Geometry: final body of the model. Coordinates: model frame, mm. A direction names the side the tool comes from. Give positions to 0.01 mm unless a question says otherwise; leave off trailing zeros. Order: outer loops, then holes, each group sorted by start corner. A loop starts at its lowest first (then second) coordinate and runs counter-clockwise, first axis right, second up. Notation, with made-up numbers: M 10.25,27.5 L 38.25,27.5 A19 ccw 38.25,36.5 Z; hole C 88.5,-29.75 d11. An arc over 180 degrees is marked long. One line per item, written item: value. Start each with the question number.
```python
from build123d import *

# Parameters (mm, degrees)
SKETCH1_R                    = 6.349999995
SKETCH1_R_2                  = 2.75
SKETCH1_R_3                  = 2.999999999
SKETCH1_R_4                  = 20
BOSS_EXTRUDE1_DEPTH          = 4.7625
FILLET1_R                    = 5.08
M5_TAPPED_HOLE1_D            = 4.2
M5_TAPPED_HOLE1_DEPTH        = 14
M5_TAPPED_HOLE1_TIP          = 1.2618073
F_3_0_3_DIAMETER_HOLE1_D     = 3
F_3_0_3_DIAMETER_HOLE1_DEPTH = 25.4
F_3_0_3_DIAMETER_HOLE1_TIP   = 0.901290929


with BuildPart() as part:
    # Sketch1 → Boss-Extrude1 (new body)
    # profile 1 of 6: a face of its own
    with BuildSketch(Plane.XY):
        Polygon((0, 57.15), (0, 0), (-8.945, -2.86), (-8.945, -40), (8.575, -40), (48.575, -40), (57.15, 0), (57.15, 57.15), align=None)
        with Locations(Location((-0.185, -21.43, 0), (0, 0, 180))):
            Circle(SKETCH1_R, mode=Mode.SUBTRACT)
        with Locations((4.953, 4.989071325)):
            Circle(SKETCH1_R_2, mode=Mode.SUBTRACT)
        with Locations(Location((28.575, -31.5, 0), (0, 0, 180))):
            Circle(SKETCH1_R_3, mode=Mode.SUBTRACT)
        with Locations(Location((28.575, -11.5, 0), (0, 0, 180))):
            Circle(SKETCH1_R_3, mode=Mode.SUBTRACT)
        with Locations((52.197, 4.989071325)):
            Circle(SKETCH1_R_2, mode=Mode.SUBTRACT)
        with Locations((4.953, 52.233071325)):
            Circle(SKETCH1_R_2, mode=Mode.SUBTRACT)
        with Locations(Location((28.575, 28.575, 0), (0, 0, 180))):
            Circle(SKETCH1_R_4, mode=Mode.SUBTRACT)
        with Locations((52.197, 52.197)):
            Circle(SKETCH1_R_2, mode=Mode.SUBTRACT)
    # profile 2 of 6: a face of its own
    with BuildSketch(Plane.XY):
        Polygon((0, 57.15), (0, 0), (-8.945, -2.86), (-8.945, -40), (8.575, -40), (48.575, -40), (57.15, 0), (57.15, 57.15), align=None)
        with Locations(Location((-0.185, -21.43, 0), (0, 0, 180))):
            Circle(SKETCH1_R, mode=Mode.SUBTRACT)
        with Locations((4.953, 4.989071325)):
            Circle(SKETCH1_R_2, mode=Mode.SUBTRACT)
        with Locations(Location((28.575, -31.5, 0), (0, 0, 180))):
            Circle(SKETCH1_R_3, mode=Mode.SUBTRACT)
        with Locations(Location((28.575, -11.5, 0), (0, 0, 180))):
            Circle(SKETCH1_R_3, mode=Mode.SUBTRACT)
        with Locations((52.197, 4.989071325)):
            Circle(SKETCH1_R_2, mode=Mode.SUBTRACT)
        with Locations((4.953, 52.233071325)):
            Circle(SKETCH1_R_2, mode=Mode.SUBTRACT)
        with Locations(Location((28.575, 28.575, 0), (0, 0, 180))):
            Circle(SKETCH1_R_4, mode=Mode.SUBTRACT)
        with Locations((52.197, 52.197)):
            Circle(SKETCH1_R_2, mode=Mode.SUBTRACT)
    # profile 3 of 6: a face of its own
    with BuildSketch(Plane.XY):
        with Locations((4.953, 52.233071325)):
            Circle(SKETCH1_R_2)
    # profile 4 of 6: a face of its own
    with BuildSketch(Plane.XY):
        with Locations((52.197, 52.197)):
            Circle(SKETCH1_R_2)
    # profile 5 of 6: a face of its own
    with BuildSketch(Plane.XY):
        with Locations((4.953, 4.989071325)):
            Circle(SKETCH1_R_2)
    # profile 6 of 6: a face of its own
    with BuildSketch(Plane.XY):
        with Locations((52.197, 4.989071325)):
            Circle(SKETCH1_R_2)
    extrude(amount=BOSS_EXTRUDE1_DEPTH)

    # Fillet1
    fillet1_edges = [part.edges().sort_by_distance(p)[0] for p in [
        (-8.945, -40, 2.38125),
        (-8.945, -2.86, 2.38125),
        (0, 0, 2.38125),
        (0, 57.15, 2.38125),
        (57.15, 57.15, 2.38125),
        (57.15, 0, 2.38125),
        (48.575, -40, 2.38125),
    ]]
    fillet(fillet1_edges, radius=FILLET1_R)

    # M5 Tapped Hole1
    with Locations(Plane.XY.offset(4.7625)):
        with Locations((4.953, 52.233071325), (52.197, 52.197), (52.197, 4.989071325), (4.953, 4.989071325)):
            Hole(M5_TAPPED_HOLE1_D / 2, depth=M5_TAPPED_HOLE1_DEPTH)
            with Locations((0, 0, -(M5_TAPPED_HOLE1_DEPTH + M5_TAPPED_HOLE1_TIP / 2))):  # 118° drill point
                Cone(0, M5_TAPPED_HOLE1_D / 2, M5_TAPPED_HOLE1_TIP, mode=Mode.SUBTRACT)

    # Ø3.0 (3) Diameter Hole1
    with Locations(Plane(origin=(0, 0, 0), x_dir=(-1, 0, 0), z_dir=(0, 0, -1))):
        with Locations((0.185, -30.96), (0.185, -11.9)):
            Hole(F_3_0_3_DIAMETER_HOLE1_D / 2, depth=F_3_0_3_DIAMETER_HOLE1_DEPTH)
            with Locations((0, 0, -(F_3_0_3_DIAMETER_HOLE1_DEPTH + F_3_0_3_DIAMETER_HOLE1_TIP / 2))):  # 118° drill point
                Cone(0, F_3_0_3_DIAMETER_HOLE1_D / 2, F_3_0_3_DIAMETER_HOLE1_TIP, mode=Mode.SUBTRACT)


solid = part.part
```
Q1. Ray query, line 1 along Y through (x, z) = (-0.5, 0.35); line 2 along X through (y, z) = (-11.5, 3.05) (3 decimals); line 3 along Y through (x, z) = (35, 3.5). Return the intervals inside material, ascending. Write a range as [from, to].
Q2. Mould query, pull axis Y, two halves, no side actions, for faces 3 (the face through (53.183, -18.504, 2.348)), 4 (the face through (29, 57.15, 2)), 5 (the face through (10.1, 36.24, 2.35)). Classes: +Y half, -Y half, draft (parallel to the pull), parting line (faces both ways), or undercut.
Q3. Section query C-C on z = 1.9. Give the number of separate pieces and of enclosed holes in the cut face, and give its area (3 significant figures).
Q4. Section query B-B on x = 36. Return loops of the section in (y, z), and give its area (3 significant figures).
Q5. Contact query for a flat-ended pin moving along its axis: pin 1 (2.5 mm diameter, centred on x = 52.2, y = 4.99, fed in from +Z). Output: stop coordinate, or through.
Q6. Section query D-D on y = -5.5. Return loops of the section in (x, z), and give its area (3 significant figures).
Q7. Set-up query: faces 1 (the face through (0, 28, 2)), 2 (the face through (3.824, 6.76, 2.348)). Return all of +Z, -Z, +X, -X, +Y, -Y with unobstructed straight access to the full face (end or side cutting, diameter ignored); none if empty.
Results below:
1. line 1: [-40, -32.43], [-29.49, -27.77], [-15.09, -13.37], [-10.43, 1.51]
1. line 2: [-8.945, -1.631], [1.261, 25.575], [31.575, 54.685]
1. line 3: [-40, 9.64], [47.51, 57.15]
2. face 3: -Y half
2. face 4: +Y half
2. face 5: undercut
3. separate pieces: 1
3. enclosed holes: 10
3. area: 4,200 mm2
4. outline: M -40,0 L 10,0 L 10,4.76 L -40,4.76 Z; M 47.15,0 L 57.15,0 L 57.15,4.76 L 47.15,4.76 Z
4. area: 286 mm2
5. pin 1: through
6. outline: M -8.83,0 L 55.97,0 L 55.97,4.76 L -8.83,4.76 Z
6. area: 309 mm2
7. face 1: +Z, -Z, -X, +Y
7. face 2: +Z, -Z
